Verification items for the finished model (mm, model axes). A direction names the side the tool comes from. Give positions to 0.01 mm unless a question says otherwise; leave off trailing zeros. Write each loop counter-clockwise with the first axis right and the second up, starting at its lowest first coordinate (ties: lowest second). Pieces come first, ordered by that corner, then holes.
Autodesk Inventor part; units mm, degrees
ref_plane "Work Plane1" through (19.65, 0, 20.2) normal (0, 0, 1) x (1, 0, 0)
ref_plane "Work Plane2" through (15.15, 0, 0) normal (0, -1, 0) x (1, 0, 0)
ref_plane "YZ Plane" through (0, 0, 0) normal (1, 0, 0) x (0, 1, 0)
sketch "Sketch1" plane through (0, 0, 0) normal (0, 0, 1) x (1, 0, 0)
  circle A0 centre (-17.4, 0) radius 1.5
  line L0 (0, 7.9375) -> (0, -7.1814) construction
  line L1 (-8.2631, 0) -> (10.6068, 0) construction
  line L2 (-19.65, 2.25) -> (-15.15, 2.25)
  line L3 (-15.15, 2.25) -> (-15.15, -2.25)
  line L4 (-15.15, -2.25) -> (-19.65, -2.25)
  line L5 (-19.65, -2.25) -> (-19.65, 2.25)
  line L6 (-19.65, 2.25) -> (-15.15, -2.25) construction
  line L7 (-15.15, 2.25) -> (-19.65, -2.25) construction
  circle A1 centre (17.4, 0) radius 1.5
  line L8 (19.65, 2.25) -> (15.15, 2.25)
  line L9 (15.15, 2.25) -> (15.15, -2.25)
  line L10 (15.15, -2.25) -> (19.65, -2.25)
  line L11 (19.65, -2.25) -> (19.65, 2.25)
  line L12 (19.65, 2.25) -> (15.15, -2.25) construction
  line L13 (15.15, 2.25) -> (19.65, -2.25) construction
  point P0 (0, 0)
  dimension "d0" = 3
  dimension "d1" = 17.4
  dimension "d2" = 4.5
  dimension "d3" = 4.5
extrude "Extrusion1" add sketch "Sketch1" along normal blind 20.2 contours A0 | L2 L3 L4 L5 | A1 | L11 L10 L9 L8
extrude "Extrusion2" cut sketch "Sketch1" along normal blind 22.2 contours A0 | A1
ref_plane "Work Plane1" through (19.65, 0, 20.2) normal (0, 0, 1) x (1, 0, 0)
sketch "Sketch2" plane through (19.65, 0, 20.2) normal (0, 0, 1) x (1, 0, 0)
  line L0 (-39.3, 2.25) -> (-39.3, -2.25)
  line L1 (0, -2.25) -> (0, 2.25)
  line L2 (-39.3, 2.25) -> (0, 2.25)
  line L3 (0, 2.25) -> (0, -2.25)
  line L4 (0, -2.25) -> (-39.3, -2.25)
  line L5 (-39.3, -2.25) -> (-39.3, 2.25)
  point P0 (-19.65, 0)
extrude "Extrusion3" add sketch "Sketch2" along normal blind 2
ref_plane "Work Plane2" through (15.15, 0, 0) normal (0, -1, 0) x (1, 0, 0)
sketch "Sketch5" plane through (15.15, 0, 0) normal (0, -1, 0) x (1, 0, 0)
  line L0 (0, 20.2) -> (-30.3, 20.2)
  line L1 (-30.3, 20.2) -> (-25.3, 20.2)
  line L2 (-30.3, 20.2) -> (-30.3, 15.2)
  line L3 (-30.3, 0) -> (-30.3, 20.2)
  line L4 (-30.3, 15.2) -> (-25.3, 20.2)
  line L5 (0, 0) -> (0, 20.2)
  line L6 (0, 20.2) -> (-5, 20.2)
  line L7 (-5, 20.2) -> (0, 15.2)
  line L8 (0, 15.2) -> (0, 20.2)
  point P0 (-15.15, 0)
  dimension "d10" = 5
  dimension "d11" = 5
  dimension "d12" = 5
extrude "Extrusion4" add sketch "Sketch5" along normal mid plane 4.5
sketch "Sketch6" plane through (19.65, 0, 22.2) normal (0, 0, 1) x (1, 0, 0)
  circle A0 centre (-37.05, 0) radius 1.5
  circle A1 centre (-37.05, 0) radius 1.5
  circle A2 centre (-2.25, 0) radius 1.5
  circle A3 centre (-2.25, 0) radius 1.5
  point P0 (-19.65, 0)
extrude "Extrusion5" cut sketch "Sketch6" against normal blind 2
thread "Thread1"
thread "Thread2"
sketch "Sketch7" plane through (19.65, -2.25, 0) normal (1, 0, 0) x (0, 0, -1)
  circle A0 centre (-6, 2.25) radius 1
  line L0 (0, 0) -> (0, 4.5)
  circle A1 centre (-18, 2.25) radius 1
  point P0 (0, 2.25)
  point P1 (0, 2.25)
  dimension "d21" = 2
  dimension "d22" = 6
  dimension "d23" = 2
  dimension "d24" = 12
extrude "Extrusion6" cut sketch "Sketch7" against normal blind 40
properties part number "Tiang 1_3DPrint"
Item 1: Set-up check for faces 1 (the face through (-15.6, 0, 7)), 2 (the face through (13.17, 1.03, 17.18)): record each of +Z, -Z, +X, -X, +Y, -Y from which the full face is reachable in a straight line by a thin tool's end or side.
Answer key:
face 1: +X, -X
face 2: -Z, +Y, -Y
Item 2: Sectioned sample at A-A on z = 12.25. Record the cut outline in (x, y).
Answer key:
outline: (-19.65, -2.25) - (-15.15, -2.25) - (-15.15, 2.25) - (-19.65, 2.25) - close; (15.15, -2.25) - (19.65, -2.25) - (19.65, 2.25) - (15.15, 2.25) - close; hole circle Ø3 at (-17.4, 0); hole circle Ø3 at (17.4, 0)
Item 3: Scan lines: line 1 along Z through (x, y) = (19.1, 0); line 2 along Y through (x, z) = (19.4, 18); line 3 along X through (y, z) = (1.1, 7.5). Record each from-to range of solid material in increasing order.
Answer key:
line 1: z = 0 to 5, 7 to 17, 19 to 22.2
line 2: y = -2.25 to -1, 1 to 2.25
line 3: x = -19.65 to -18.42, -16.38 to -15.15, 15.15 to 16.38, 18.42 to 19.65
Item 4: Depth check by flat-ended pin: pin 1 (1.3 mm diameter, centred on x = -1, y = 0.5, fed in from -Z). Enter the tip coordinate at first touch or a pass-through.
Answer key:
pin 1: stops at z = 20.2
Item 5: Release check for a two-part mould opening along X. For faces 3 (the face through (19.65, 0, 11)), 4 (the face through (-14, 0, 19)), 5 (the face through (-13.24, 1.03, 17.11)) record: released by +X, released by -X, zero draft, split by the parting line, or undercut.
Answer key:
face 3: released by +X
face 4: zero draft
face 5: undercut
Item 6: Sectioned sample at B-B on x = -17.4. Record the cut outline in (y, z).
Answer key:
outline: (-2.25, 0) - (-1.5, 0) - (-1.5, 22.2) - (-2.25, 22.2) - close; (1.5, 0) - (2.25, 0) - (2.25, 22.2) - (1.5, 22.2) - close
Item 7: Sectioned sample at C-C on z = 18. Record the cut outline in (x, y).
Answer key:
outline: (-19.65, -2.25) - (-12.35, -2.25) - (-12.35, -1) - (-16.28, -1) arc R1.5 cw to (-18.52, -1) - (-19.65, -1) - close; (-19.65, 1) - (-18.52, 1) arc R1.5 cw to (-16.28, 1) - (-12.35, 1) - (-12.35, 2.25) - (-19.65, 2.25) - close; (12.35, -2.25) - (19.65, -2.25) - (19.65, -1) - (18.52, -1) arc R1.5 cw to (16.28, -1) - (12.35, -1) - close; (12.35, 1) - (16.28, 1) arc R1.5 cw to (18.52, 1) - (19.65, 1) - (19.65, 2.25) - (12.35, 2.25) - close
Item 8: Sectioned sample at D-D on y = 0. State how many separate pieces and enclosed holes the cut face has, then the cut area to 3 significant figures.
Answer key:
separate pieces: 11
enclosed holes: 0
area: 129 mm2
